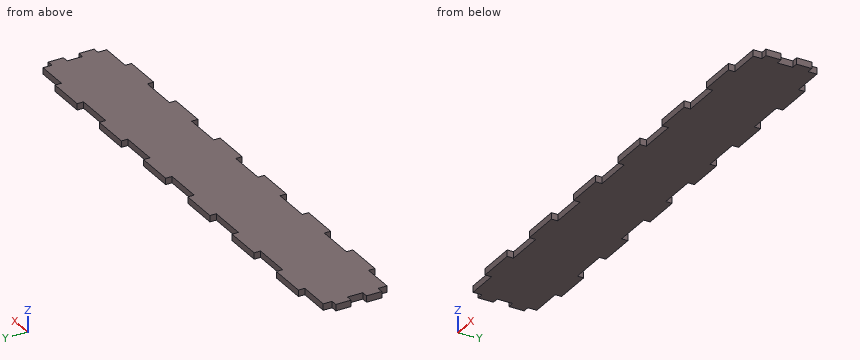
from build123d import *

# Parameters (mm, degrees)
ESQUISSE1_W                = 390
ESQUISSE1_H                = 60
BOSS_EXTRU_1_DEPTH         = 5
ESQUISSE2_W                = 30
ESQUISSE2_H                = 5
ENL_V_MAT_EXTRU_1_DEPTH    = 5
R_P_TITION_LIN_AIRE1_COUNT = 7
R_P_TITION_LIN_AIRE1_PITCH = 60
ESQUISSE3_W                = 5
ESQUISSE3_H                = 12
ENL_V_MAT_EXTRU_2_DEPTH    = 5
R_P_TITION_LIN_AIRE2_COUNT = 3
R_P_TITION_LIN_AIRE2_PITCH = 24
SYM_TRIE1_COPY_1_SKETCH_W  = 5
SYM_TRIE1_COPY_1_SKETCH_H  = 12
SYM_TRIE1_COPY_1_DEPTH     = 5
SYM_TRIE1_COPY_2_SKETCH_W  = 5
SYM_TRIE1_COPY_2_SKETCH_H  = 12
SYM_TRIE1_COPY_2_DEPTH     = 5
SYM_TRIE2_COPY_1_SKETCH_W  = 30
SYM_TRIE2_COPY_1_SKETCH_H  = 5
SYM_TRIE2_COPY_1_DEPTH     = 5
SYM_TRIE2_COPY_2_SKETCH_W  = 30
SYM_TRIE2_COPY_2_SKETCH_H  = 5
SYM_TRIE2_COPY_2_DEPTH     = 5
SYM_TRIE2_COPY_3_SKETCH_W  = 30
SYM_TRIE2_COPY_3_SKETCH_H  = 5
SYM_TRIE2_COPY_3_DEPTH     = 5
SYM_TRIE2_COPY_4_SKETCH_W  = 30
SYM_TRIE2_COPY_4_SKETCH_H  = 5
SYM_TRIE2_COPY_4_DEPTH     = 5
SYM_TRIE2_COPY_5_SKETCH_W  = 30
SYM_TRIE2_COPY_5_SKETCH_H  = 5
SYM_TRIE2_COPY_5_DEPTH     = 5
SYM_TRIE2_COPY_6_SKETCH_W  = 30
SYM_TRIE2_COPY_6_SKETCH_H  = 5
SYM_TRIE2_COPY_6_DEPTH     = 5


with BuildPart() as part:
    # Esquisse1 → Boss.-Extru.1 (new body)
    with BuildSketch(Plane.XY):
        with Locations((195, -30)):
            Rectangle(ESQUISSE1_W, ESQUISSE1_H)
    extrude(amount=BOSS_EXTRU_1_DEPTH)

    # Esquisse2 → Enlèv. mat.-Extru.1 (cut)
    with BuildSketch(Plane.XY.offset(5)):
        with Locations((15, -57.5)):
            Rectangle(ESQUISSE2_W, ESQUISSE2_H)
    enl_v_mat_extru_1 = extrude(amount=-ENL_V_MAT_EXTRU_1_DEPTH, mode=Mode.SUBTRACT)

    # Répétition linéaire1: Enlèv. mat.-Extru.1 ×7
    with Locations(*[(i * R_P_TITION_LIN_AIRE1_PITCH, 0, 0) for i in range(1, R_P_TITION_LIN_AIRE1_COUNT)]):
        add(enl_v_mat_extru_1, mode=Mode.SUBTRACT)

    # Esquisse3 → Enlèv. mat.-Extru.2 (cut)
    with BuildSketch(Plane.XY.offset(5)):
        with Locations((2.5, -54)):
            Rectangle(ESQUISSE3_W, ESQUISSE3_H)
    enl_v_mat_extru_2 = extrude(amount=-ENL_V_MAT_EXTRU_2_DEPTH, mode=Mode.SUBTRACT)

    # Répétition linéaire2: Enlèv. mat.-Extru.2 ×3
    with Locations(*[(0, i * R_P_TITION_LIN_AIRE2_PITCH, 0) for i in range(1, R_P_TITION_LIN_AIRE2_COUNT)]):
        add(enl_v_mat_extru_2, mode=Mode.SUBTRACT)

    # Symétrie1: Enlèv. mat.-Extru.2 across plane
    add(enl_v_mat_extru_2.mirror(Plane.ZY.offset(-195)), mode=Mode.SUBTRACT)

    # Symétrie1 copy 1 sketch → Symétrie1 copy 1 (cut)
    with BuildSketch(Plane(origin=(390, 24, 5), x_dir=(-1, 0, 0), z_dir=(0, 0, 1))):
        with Locations((2.5, 54)):
            Rectangle(SYM_TRIE1_COPY_1_SKETCH_W, SYM_TRIE1_COPY_1_SKETCH_H)
    extrude(amount=-SYM_TRIE1_COPY_1_DEPTH, mode=Mode.SUBTRACT)

    # Symétrie1 copy 2 sketch → Symétrie1 copy 2 (cut)
    with BuildSketch(Plane(origin=(390, 48, 5), x_dir=(-1, 0, 0), z_dir=(0, 0, 1))):
        with Locations((2.5, 54)):
            Rectangle(SYM_TRIE1_COPY_2_SKETCH_W, SYM_TRIE1_COPY_2_SKETCH_H)
    extrude(amount=-SYM_TRIE1_COPY_2_DEPTH, mode=Mode.SUBTRACT)

    # Symétrie2: Enlèv. mat.-Extru.1 across plane
    add(enl_v_mat_extru_1.mirror(Plane(origin=(0, -30, 0), x_dir=(0, 0, 1), z_dir=(0, -1, 0))), mode=Mode.SUBTRACT)

    # Symétrie2 copy 1 sketch → Symétrie2 copy 1 (cut)
    with BuildSketch(Plane(origin=(60, -60, 5), x_dir=(1, 0, 0), z_dir=(0, 0, 1))):
        with Locations((15, 57.5)):
            Rectangle(SYM_TRIE2_COPY_1_SKETCH_W, SYM_TRIE2_COPY_1_SKETCH_H)
    extrude(amount=-SYM_TRIE2_COPY_1_DEPTH, mode=Mode.SUBTRACT)

    # Symétrie2 copy 2 sketch → Symétrie2 copy 2 (cut)
    with BuildSketch(Plane(origin=(120, -60, 5), x_dir=(1, 0, 0), z_dir=(0, 0, 1))):
        with Locations((15, 57.5)):
            Rectangle(SYM_TRIE2_COPY_2_SKETCH_W, SYM_TRIE2_COPY_2_SKETCH_H)
    extrude(amount=-SYM_TRIE2_COPY_2_DEPTH, mode=Mode.SUBTRACT)

    # Symétrie2 copy 3 sketch → Symétrie2 copy 3 (cut)
    with BuildSketch(Plane(origin=(180, -60, 5), x_dir=(1, 0, 0), z_dir=(0, 0, 1))):
        with Locations((15, 57.5)):
            Rectangle(SYM_TRIE2_COPY_3_SKETCH_W, SYM_TRIE2_COPY_3_SKETCH_H)
    extrude(amount=-SYM_TRIE2_COPY_3_DEPTH, mode=Mode.SUBTRACT)

    # Symétrie2 copy 4 sketch → Symétrie2 copy 4 (cut)
    with BuildSketch(Plane(origin=(240, -60, 5), x_dir=(1, 0, 0), z_dir=(0, 0, 1))):
        with Locations((15, 57.5)):
            Rectangle(SYM_TRIE2_COPY_4_SKETCH_W, SYM_TRIE2_COPY_4_SKETCH_H)
    extrude(amount=-SYM_TRIE2_COPY_4_DEPTH, mode=Mode.SUBTRACT)

    # Symétrie2 copy 5 sketch → Symétrie2 copy 5 (cut)
    with BuildSketch(Plane(origin=(300, -60, 5), x_dir=(1, 0, 0), z_dir=(0, 0, 1))):
        with Locations((15, 57.5)):
            Rectangle(SYM_TRIE2_COPY_5_SKETCH_W, SYM_TRIE2_COPY_5_SKETCH_H)
    extrude(amount=-SYM_TRIE2_COPY_5_DEPTH, mode=Mode.SUBTRACT)

    # Symétrie2 copy 6 sketch → Symétrie2 copy 6 (cut)
    with BuildSketch(Plane(origin=(360, -60, 5), x_dir=(1, 0, 0), z_dir=(0, 0, 1))):
        with Locations((15, 57.5)):
            Rectangle(SYM_TRIE2_COPY_6_SKETCH_W, SYM_TRIE2_COPY_6_SKETCH_H)
    extrude(amount=-SYM_TRIE2_COPY_6_DEPTH, mode=Mode.SUBTRACT)


solid = part.part
Source: CAD feature listing. Evaluate the final solid. Frame: model axes, mm. Coordinates: 2 decimals unless noted, no trailing zeros. Order: outer loops, then holes, each group sorted by start corner. A loop starts at its lowest first (then second) coordinate and runs counter-clockwise, first axis right, second up.
Item 1: Cut plane A-A (y = -31). Return loops of the section in (x, z), plus the area to 3 significant figures.
Output values:
outline: (5, 0) - (385, 0) - (385, 5) - (5, 5) - close
area: 1,900 mm2
Item 2: First-contact query: P1, Ø2.5, axis at y = -2, z = 1.5, coming from the +X side; P2, Ø2.5, axis at x = 134.5, z = 3, coming from the -Y side; P3, Ø1.5, axis at y = -58, z = 3.5, coming from the -X side. Flat tips, straight axial feed; report the tip coordinate or a pass-through.
Output values:
P1: stops at x = 360
P2: stops at y = -55
P3: stops at x = 30
Item 3: Material intervals for line 1 (X direction, y = -57, z = 1.9); line 2 (X direction, y = -25, z = 2.6); line 3 (Y direction, x = 66, z = 0.3), sorted ascending.
Output values:
line 1: x = 30 to 60, 90 to 120, 150 to 180, 210 to 240, 270 to 300, 330 to 360
line 2: x = 5 to 385
line 3: y = -55 to -5
Item 4: Cut plane B-B (x = 83). Return loops of the section in (y, z), plus the area to 3 significant figures.
Output values:
outline: (-55, 0) - (-5, 0) - (-5, 5) - (-55, 5) - close
area: 250 mm2
